Model file for the job. Use its own axes, mm. A direction names the side the tool comes from. Round coordinates to 2 decimals unless told otherwise and drop trailing zeros. Write each loop counter-clockwise with the first axis right and the second up, starting at its lowest first coordinate (ties: lowest second). Pieces come first, ordered by that corner, then holes. Notation, with made-up numbers: (47.5, 71) - (95.5, 71) arc R13 cw to (95.5, 85) - close; hole circle Ø9 at (-8, 14). An arc over 180 degrees is marked (long way). Answer as a JSON object with one key per item and string values. Group by question number.
from build123d import *

# Parameters (mm, degrees)
SCHIZZO1_R                   = 4
ESTRUSIONE_ESTRUSIONE1_DEPTH = 5


with BuildPart() as part:
    # Schizzo1 → Estrusione-Estrusione1 (new body)
    with BuildSketch(Plane.XY):
        with BuildLine():
            Line((18.440051647, 15), (123.269745712, 15))
            Line((123.269745712, 15), (142.855666239, 6.935068156))
            ThreePointArc((142.855666239, 6.935068156), (146.82520143, -3.10911972), (136.641644665, -6.706075562))
            Line((136.641644665, -6.706075562), (117.260230363, 3))
            Line((117.260230363, 3), (21.046177465, 3))
            Line((21.046177465, 3), (2.488742023, -5.459502096))
            ThreePointArc((2.488742023, -5.459502096), (-5.459502096, -2.488742023), (-2.488742023, 5.459502096))
            Line((-2.488742023, 5.459502096), (18.440051647, 15))
        make_face()
        Circle(SCHIZZO1_R, mode=Mode.SUBTRACT)
        with Locations((140, 0)):
            Circle(SCHIZZO1_R, mode=Mode.SUBTRACT)
    extrude(amount=ESTRUSIONE_ESTRUSIONE1_DEPTH)


solid = part.part
(1) Flat gauge pins, fed straight in: pin 1 (1.5 mm diameter, centred on x = 57.5, z = 1.5, fed in from -Y); pin 2 (3 mm diameter, centred on y = -3.5, z = 2.5, fed in from +X); pin 3 (1 mm diameter, centred on x = 128, z = 2, fed in from -Y). Where does each tip first touch, or does it go through?
(2) Slice it at A-A (z = 2.75). Write the cut outline in (x, y).
(3) Slice it at B-B (x = 140). Write the cut outline in (y, z).
(4) Drill centre lines: line 1 (X direction, y = -2.75, z = 3.85); line 2 (X direction, y = 0.5, z = 0.3); line 3 (Y direction, x = 99, z = 2.85). Where is each one in solid material? Low to high. Write a range as from..to.
(5) 3-axis set-ups, long thin cutter, end or side, ignore diameter. For faces 5 (the flat face through (127.087, -1.921, 2.465)), 6 (the cylindrical face through (-0.867, -3.905, 2.465)): which of +Z, -Z, +X, -X, +Y, -Y reach the whole face in a straight line?
(6) Slice it at C-C (y = 0). Write the cut outline in (x, z).
(7) Slice it at D-D (x = 23). Write the cut outline in (y, z), then the cut area to 3 significant figures.
(8) Pull direction Y, two halves, no side cores. Call faces 1 (the cylindrical face through (143.815, 1.201, 2.465)), 2 (the flat face through (70, 3, 2)), 3 (the flat face through (7.829, 10.163, 2.465)), 4 (the cylindrical face through (146.893, -2.955, 2.465)): pulls with the +Y half, pulls with the -Y half, needs draft (parallel to the pull), parting line crosses it, or undercut.
Answer:
{
 "1": {"pin 1": "y = 3", "pin 2": "x = 147.23", "pin 3": "y = -2.63"},
 "2": {"outline": "(-2.49, 5.46) arc R6 ccw to (2.49, -5.46) - (21.05, 3) - (117.26, 3) - (136.64, -6.71) arc R7.5 ccw (long way) to (142.86, 6.94) - (123.27, 15) - (18.44, 15) - close; hole circle Ø8 at (0, 0); hole circle Ø8 at (140, 0)"},
 "3": {"outline": "(-7.5, 0) - (-4, 0) - (-4, 5) - (-7.5, 5) - close; (4, 0) - (8.11, 0) - (8.11, 5) - (4, 5) - close"},
 "4": {"line 1": "-5.33..-2.9, 2.9..8.43, 128.74..137.1, 142.9..146.98", "line 2": "-5.98..-3.97, 3.97..15.56, 122.25..136.03, 143.97..147.48", "line 3": "3..15"},
 "5": {"face 5": "+Z, -Z, -Y", "face 6": "+Z, -Z"},
 "6": {"outline": "(-6, 0) - (-4, 0) - (-4, 5) - (-6, 5) - close; (4, 0) - (14.47, 0) - (14.47, 5) - (4, 5) - close; (123.25, 0) - (136, 0) - (136, 5) - (123.25, 5) - close; (144, 0) - (147.5, 0) - (147.5, 5) - (144, 5) - close"},
 "7": {"outline": "(3, 0) - (15, 0) - (15, 5) - (3, 5) - close", "area": "60.0 mm²"},
 "8": {"face 1": "undercut", "face 2": "pulls with the -Y half", "face 3": "pulls with the +Y half", "face 4": "parting line crosses it"}
}
